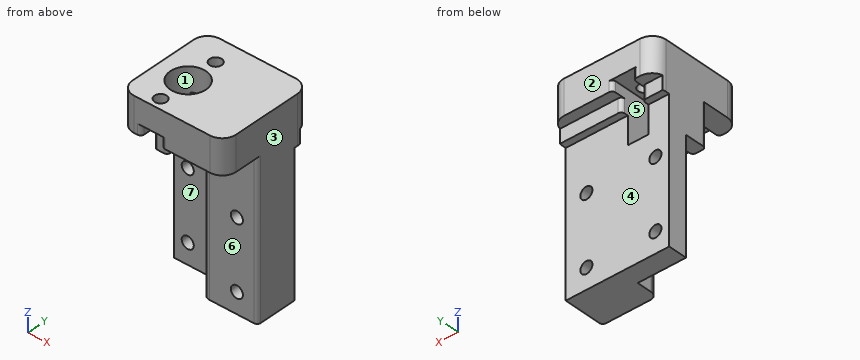
from build123d import *

# Parameters (mm, degrees)
PAD001_DEPTH      = 16
PAD001_DEPTH_BACK = 16
SKETCH014_W       = 15
SKETCH014_H       = 6
POCKET_DEPTH      = 28.001
SKETCH012_R       = 5.15
POCKET001_DEPTH   = 55.001
SKETCH013_R       = 1.75
POCKET002_DEPTH   = 7
SKETCH008_W       = 7.407674
SKETCH008_H       = 16
POCKET003_DEPTH   = 33
SKETCH007_R       = 1.75
POCKET004_DEPTH   = 17.001
SKETCH015_W       = 50.47
SKETCH015_H       = 40
POCKET005_DEPTH   = 2
SKETCH016_W       = 51.98
SKETCH016_H       = 14.53
POCKET006_DEPTH   = 55.001
FILLET_R          = 4
FILLET001_R       = 1
FILLET002_R       = 2
FILLET003_R       = 1
FILLET004_R       = 1
FILLET005_R       = 1
FILLET006_R       = 1


with BuildPart() as part:
    # Sketch005 → Pad001 (new body, two sides)
    with BuildSketch(Plane.YZ) as pad001_sk:
        Polygon((0, -20), (0, 25), (3, 25), (3, 35), (-25, 35), (-25, 25), (-14, 25), (-14, -20), align=None)
    extrude(amount=PAD001_DEPTH)
    extrude(pad001_sk.sketch, amount=-PAD001_DEPTH_BACK)

    # Sketch014 (on Face5 of Pad001) → Pocket (cut, through all)
    with BuildSketch(Plane(origin=(0, -25, 0), x_dir=(0, 0, -1), z_dir=(0, -1, 0))):
        with Locations((-20.5, -5)):
            Rectangle(SKETCH014_W, SKETCH014_H)
    extrude(amount=-POCKET_DEPTH, mode=Mode.SUBTRACT)

    # Sketch012 → Pocket001 (cut, through all)
    with BuildSketch(Plane(origin=(0, 0, 35), x_dir=(0, -1, 0), z_dir=(0, 0, 1))):
        with Locations((13, -5)):
            Circle(SKETCH012_R)
    extrude(amount=-POCKET001_DEPTH, mode=Mode.SUBTRACT)

    # Sketch013 → Pocket002 (cut)
    with BuildSketch(Plane(origin=(0, 0, 35), x_dir=(0, -1, 0), z_dir=(0, 0, 1))):
        with Locations((4, -5)):
            Circle(SKETCH013_R)
        with Locations((22, -5)):
            Circle(SKETCH013_R)
    extrude(amount=-POCKET002_DEPTH, mode=Mode.SUBTRACT)

    # Sketch008 (on Face9 of Pocket002) → Pocket003 (cut)
    with BuildSketch(Plane.YX.offset(20)):
        with Locations((-11.203837, -8)):
            Rectangle(SKETCH008_W, SKETCH008_H)
    extrude(amount=-POCKET003_DEPTH, mode=Mode.SUBTRACT)

    # Sketch007 (on Face21 of Pocket003) → Pocket004 (cut, through all)
    with BuildSketch(Plane(origin=(0, -14, 0), x_dir=(0, 0, -1), z_dir=(0, -1, 0))):
        with Locations((-6, 10)):
            Circle(SKETCH007_R)
        with Locations((14, 10)):
            Circle(SKETCH007_R)
        with Locations((-6, -10)):
            Circle(SKETCH007_R)
        with Locations((14, -10)):
            Circle(SKETCH007_R)
    extrude(amount=-POCKET004_DEPTH, mode=Mode.SUBTRACT)

    # Sketch015 (on Face1 of Pocket004) → Pocket005 (cut)
    with BuildSketch(Plane.ZX):
        with Locations((-4.235, 0)):
            Rectangle(SKETCH015_W, SKETCH015_H)
    extrude(amount=-POCKET005_DEPTH, mode=Mode.SUBTRACT)

    # Sketch016 (on Face11 of Pocket005) → Pocket006 (cut, through all)
    with BuildSketch(Plane(origin=(0, 0, 35), x_dir=(0, -1, 0), z_dir=(0, 0, 1))):
        with Locations((19.41, -21.265)):
            Rectangle(SKETCH016_W, SKETCH016_H)
    extrude(amount=-POCKET006_DEPTH, mode=Mode.SUBTRACT)

    # Fillet
    fillet_edges = [part.edges().sort_by_distance(p)[0] for p in [
        (16, -25, 30),
        (-14, -25, 30),
        (16, 3, 30),
        (-14, 3, 30),
    ]]
    fillet(fillet_edges, radius=FILLET_R)

    # Fillet001
    fillet001_edges = [part.edges().sort_by_distance(p)[0] for p in [
        (-2, -25, 26.5),
        (-8, -25, 26.5),
    ]]
    fillet(fillet001_edges, radius=FILLET001_R)

    # Fillet002
    fillet002_edges = [part.edges().sort_by_distance(p)[0] for p in [
        (0.05198, -14, 2.5),
    ]]
    fillet(fillet002_edges, radius=FILLET002_R)

    # Fillet003
    fillet003_edges = [part.edges().sort_by_distance(p)[0] for p in [
        (-14, -14, 19),
        (-10.05198, -14, 19),
    ]]
    fillet(fillet003_edges, radius=FILLET003_R)

    # Fillet004
    fillet004_edges = [part.edges().sort_by_distance(p)[0] for p in [
        (-2, 3, 26.5),
        (-8, 3, 26.5),
    ]]
    fillet(fillet004_edges, radius=FILLET004_R)

    # Fillet005
    fillet005_edges = [part.edges().sort_by_distance(p)[0] for p in [
        (-8, 0, 23),
        (-2, 0, 23),
    ]]
    fillet(fillet005_edges, radius=FILLET005_R)

    # Fillet006
    fillet006_edges = [part.edges().sort_by_distance(p)[0] for p in [
        (16, -14, 2.5),
    ]]
    fillet(fillet006_edges, radius=FILLET006_R)


solid = part.part
Work out the finished part from the listing and answer in its coordinate system (mm). Face numbers are marked on the shaded views. A direction names the side the tool comes from. Coordinates: 2 decimals unless noted, no trailing zeros. Loops run counter-clockwise (first coordinate to the right, second up) from the corner with the lowest first, then second, coordinate; pieces in that order, holes last. Notation, with made-up numbers: (24, -39.5) -> (40, -39.5) arc R20 ccw to (40, -26.5) -> close; hole circle Ø8 at (22.5, -28.5). An arc over 180 degrees is marked (long way). Write each question's results on one line, items separated by ' | '. Start each with the question number.
1) Find section B-B on y = -4. Determine the outline of the cut face in (x, z), then the cut area to 3 significant figures.
2) Find section A-A on x = 10. Determine the outline of the cut face in (y, z), then the cut area to 3 significant figures.
3) For the marked faces 4, 5, 6 and 7, determine the directions among +Z, -Z, +X, -X, +Y, -Y from which every point of the face is accessible in a straight line to the end or side of a thin tool.
4) Find section C-C on z = 19. Determine the outline of the cut face in (x, y), then the cut area to 3 significant figures.
5) Consider line 1 along X through (y, z) = (-3.65, -14); line 2 along Z through (x, y) = (8.5, -5); line 3 along X through (y, z) = (-9.75, 17) (3 decimals). Determine where each line is inside the solid, lowest interval first.
6) Flat-ended cylindrical pins translate along their axes: P1, Ø1, axis at x = -1, y = -10.5, coming from the -Z side; P2, Ø2, axis at x = 3, z = -7.5, coming from the +Y side; P3, Ø1.3, axis at y = -9, z = -7.5, coming from the -X side; P4, Ø5, axis at y = -18.5, z = 6, coming from the +X side. Find the tip coordinate at first contact, or state that the pin passes through.
7) Find section D-D on z = 6. Determine the outline of the cut face in (x, y).
8) The mould has two halves that part along Y. Classify the marked faces 1, 2 and 3: pulls with the +Y half, pulls with the -Y half, needs draft (parallel to the pull), parting line crosses it, or undercut.
Response values:
1) outline: (-14, -20) -> (16, -20) -> (16, 35) -> (-3.25, 35) -> (-3.25, 28) -> (-2, 28) -> (-2, 13) -> (-8, 13) -> (-8, 28) -> (-6.75, 28) -> (-6.75, 35) -> (-14, 35) -> close; hole circle Ø3.5 at (-10, -14); hole circle Ø3.5 at (-10, 6); hole circle Ø3.5 at (10, -14); hole circle Ø3.5 at (10, 6) | area: 1,500 mm^2
2) outline: (-25, 25) -> (-14, 25) -> (-14, 7.75) -> (-2, 7.75) -> (-2, 21) -> (0, 21) -> (0, 25) -> (3, 25) -> (3, 35) -> (-25, 35) -> close; (-14, -20) -> (-2, -20) -> (-2, -15.75) -> (-14, -15.75) -> close; (-14, -12.25) -> (-2, -12.25) -> (-2, 4.25) -> (-14, 4.25) -> close | area: 744 mm^2
3) face 4: -Z, +X, -X, +Y | face 5: +Y, -Y | face 6: -Z, +X, -X, -Y | face 7: -Z, -X, -Y
4) outline: (-14, -13) arc R1 ccw to (-13, -14) -> (-11.15, -14) arc R1 ccw to (-10.15, -13) arc R5.15 cw to (-8, -8.81) -> (-8, -2) -> (-14, -2) -> close; (-2, -8.81) arc R5.15 cw to (0.1, -12.28) arc R2 ccw to (2.08, -14) -> (15, -14) arc R1 ccw to (16, -13) -> (16, -2) -> (-2, -2) -> close | area: 270 mm^2
5) line 1: x = -14 to -11.75, -8.25 to 8.25, 11.75 to 16 | line 2: z = -20 to -14.9, -13.1 to 5.1, 6.9 to 35 | line 3: x = -14 to -8.995, -1.005 to 16
6) P1: stops at z = 13 | P2: stops at y = -2 | P3: stops at x = 0 | P4: passes through
7) outline: (-14, -7.5) -> (-11.75, -7.5) -> (-11.75, -2) -> (-14, -2) -> close; (-8.25, -7.5) -> (0, -7.5) -> (0, -11.77) arc R5.15 cw to (0.1, -12.28) arc R2 ccw to (2.08, -14) -> (8.25, -14) -> (8.25, -2) -> (-8.25, -2) -> close; (11.75, -14) -> (15, -14) arc R1 ccw to (16, -13) -> (16, -2) -> (11.75, -2) -> close
8) face 1: undercut | face 2: pulls with the +Y half | face 3: needs draft
